Source: three-view drawing plus pictorial views. Frame: mm from the lowest corner of the part. Give positions to 0.01 mm unless a question says otherwise; leave off trailing zeros. Write each loop counter-clockwise with the first axis right and the second up, starting at its lowest first coordinate (ties: lowest second). Pieces come first, ordered by that corner, then holes. Notation, with made-up numbers: (79, 79) -> (123, 79) arc R31 ccw to (123, 105) -> close; hole circle Ø1 at (50, 0.5). An arc over 180 degrees is marked (long way). Answer in a Markdown table with one row per item. Add a question column.
Item 1: Section query B-B on x = 6.25. Output: boundary loops of the cut face in (y, z), plus the area to 3 significant figures.
Item 2: Material intervals for probe 1 along Y at (x, z) = (100, 6.5); probe 2 along X at (y, z) = (172, 6.5); probe 3 along Y at (x, z) = (27.5, 6.75), sorted ascending. Write a range as from..to.
Item 3: Section query A-A on y = 100. Output: boundary loops of the cut face in (x, z).
Item 4: Section query D-D on z = 3.5. Output: boundary loops of the cut face in (x, y), plus the area to 3 significant figures.
Item 5: First-contact query: P1, Ø4, axis at y = 176, z = 3, coming from the +X side; P2, Ø13, axis at x = 193.75, y = 100, coming from the -Z side. Flat tips, straight axial feed; report the tip coordinate or a pass-through.
Item 6: Section query C-C on y = 55. Output: boundary loops of the cut face in (x, z), plus the area to 3 significant figures.
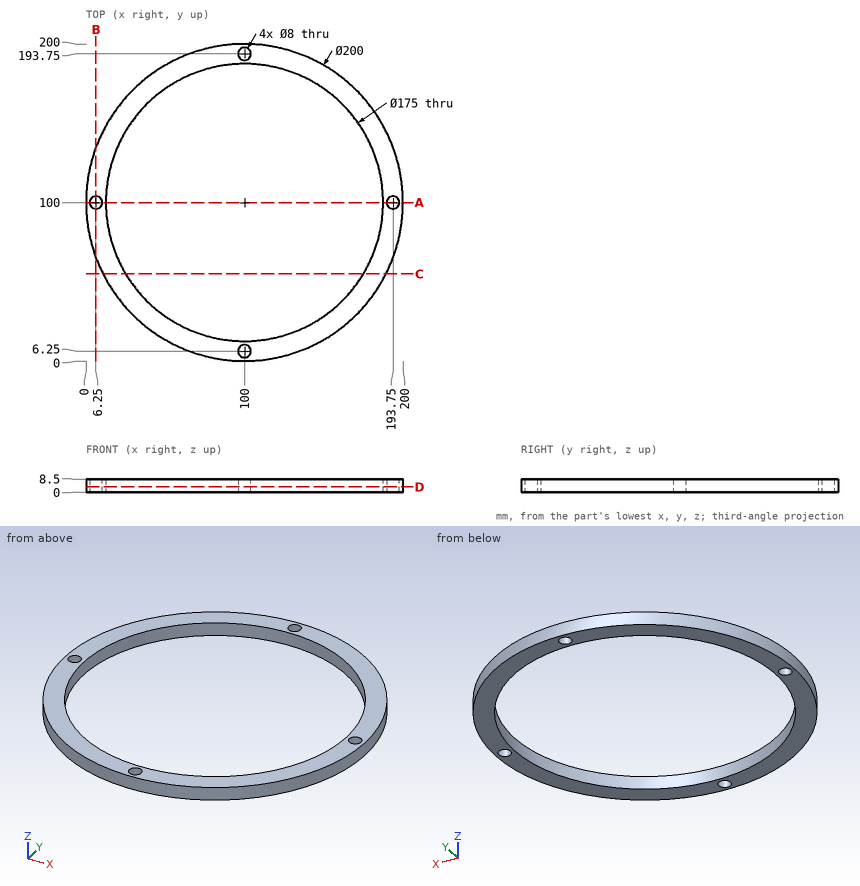
Findings below:
| question | item | result |
|---|---|---|
| 1 | outline | (65.2, 0) -> (96, 0) -> (96, 8.5) -> (65.2, 8.5) -> close; (104, 0) -> (134.8, 0) -> (134.8, 8.5) -> (104, 8.5) -> close |
| 1 | area | 524 mm^2 |
| 2 | probe 1 | y = 0..2.25, 10.25..12.5, 187.5..189.75, 197.75..200 |
| 2 | probe 2 | x = 30.6..50.28, 149.72..169.4 |
| 2 | probe 3 | y = 31.13..51.01, 148.99..168.87 |
| 3 | outline | (0, 0) -> (2.25, 0) -> (2.25, 8.5) -> (0, 8.5) -> close; (10.25, 0) -> (12.5, 0) -> (12.5, 8.5) -> (10.25, 8.5) -> close; (187.5, 0) -> (189.75, 0) -> (189.75, 8.5) -> (187.5, 8.5) -> close; (197.75, 0) -> (200, 0) -> (200, 8.5) -> (197.75, 8.5) -> close |
| 4 | outline | circle Ø200 at (100, 100); hole circle Ø8 at (6.25, 100); hole circle Ø175 at (100, 100); hole circle Ø8 at (100, 6.25); hole circle Ø8 at (100, 193.75); hole circle Ø8 at (193.75, 100) |
| 4 | area | 7,160 mm^2 |
| 5 | P1 | stops at x = 167.26 |
| 5 | P2 | stops at z = 0 |
| 6 | outline | (10.7, 0) -> (24.96, 0) -> (24.96, 8.5) -> (10.7, 8.5) -> close; (175.04, 0) -> (189.3, 0) -> (189.3, 8.5) -> (175.04, 8.5) -> close |
| 6 | area | 242 mm^2 |
